from build123d import *

# Parameters (mm, degrees)
SKETCH1_R           = 10
SKETCH1_R_2         = 40
BOSS_EXTRUDE1_DEPTH = 20
SKETCH2_W           = 119.888
SKETCH2_H           = 160
BOSS_EXTRUDE3_DEPTH = 5.08
SKETCH2_7_R         = 29.972
CUT_EXTRUDE1_DEPTH  = 257.843634424
FILLET1_R           = 9.906
FILLET2_R           = 9.906
BOSS_EXTRUDE4_DEPTH = 25.4
BOSS_EXTRUDE5_DEPTH = 25.4


with BuildPart() as part:
    # Sketch1 → Boss-Extrude1 (new body)
    with BuildSketch(Plane.XY.offset(20)):
        with BuildLine():
            Line((95, 80), (-95, 80))
            ThreePointArc((-95, 80), (-98.535533906, 78.535533906), (-100, 75))
            Line((-100, 75), (-100, -75))
            ThreePointArc((-100, -75), (-98.535533906, -78.535533906), (-95, -80))
            Line((-95, -80), (95, -80))
            Line((95, -80), (100, -80))
            Line((100, -80), (100, -75))
            Line((100, -75), (100, 75))
            Line((100, 75), (100, 80))
            Line((100, 80), (95, 80))
        make_face()
        with Locations(Location((-77.895356155, 62.316284924, 0), (0, 0, 180))):
            Circle(SKETCH1_R, mode=Mode.SUBTRACT)
        with Locations(Location((83.46, 0.37, 0), (0, 0, 180))):
            Circle(SKETCH1_R, mode=Mode.SUBTRACT)
        with Locations(Location((-77.895356155, -62.316284924, 0), (0, 0, 180))):
            Circle(SKETCH1_R, mode=Mode.SUBTRACT)
        with Locations(Location((0, 0, 0), (0, 0, 180))):
            Circle(SKETCH1_R_2, mode=Mode.SUBTRACT)
    extrude(amount=-BOSS_EXTRUDE1_DEPTH)

    # Sketch2 → Boss-Extrude3 (add)
    with BuildSketch(Plane(origin=(100, 0, 0), x_dir=(0, 0, -1), z_dir=(1, 0, 0))):
        with Locations((-79.944, 0)):
            Rectangle(SKETCH2_W, SKETCH2_H)
    extrude(amount=-BOSS_EXTRUDE3_DEPTH)

    # Sketch2_7 → Cut-Extrude1 (cut, through all)
    with BuildSketch(Plane(origin=(100, 0, 0), x_dir=(0, 0, -1), z_dir=(1, 0, 0))):
        with Locations((-100.01, 0)):
            Circle(SKETCH2_7_R)
    extrude(amount=-CUT_EXTRUDE1_DEPTH, mode=Mode.SUBTRACT)

    # Fillet1
    fillet1_edges = [part.edges().sort_by_distance(p)[0] for p in [
        (97.46, 80, 139.888),
    ]]
    fillet(fillet1_edges, radius=FILLET1_R)

    # Fillet2
    fillet2_edges = [part.edges().sort_by_distance(p)[0] for p in [
        (97.46, -80, 139.888),
    ]]
    fillet(fillet2_edges, radius=FILLET2_R)

    # Sketch4 → Boss-Extrude4 (add)
    with BuildSketch(Plane.XZ.offset(80)):
        Polygon((94.92, 129.982), (94.92, 20), (-65.1, 20), align=None)
        Polygon((82.22, 32.7), (-24.200327544, 32.7), (82.22, 105.842860042), align=None, mode=Mode.SUBTRACT)
    extrude(amount=-BOSS_EXTRUDE4_DEPTH)

    # Sketch5 → Boss-Extrude5 (add)
    with BuildSketch(Plane(origin=(0, 80, 0), x_dir=(1, 0, 0), z_dir=(0, 1, 0))):
        Polygon((94.92, -129.982), (94.92, -20), (-65.1, -20), align=None)
        Polygon((-24.200327544, -32.7), (82.22, -105.842860042), (82.22, -32.7), align=None, mode=Mode.SUBTRACT)
    extrude(amount=-BOSS_EXTRUDE5_DEPTH)


solid = part.part
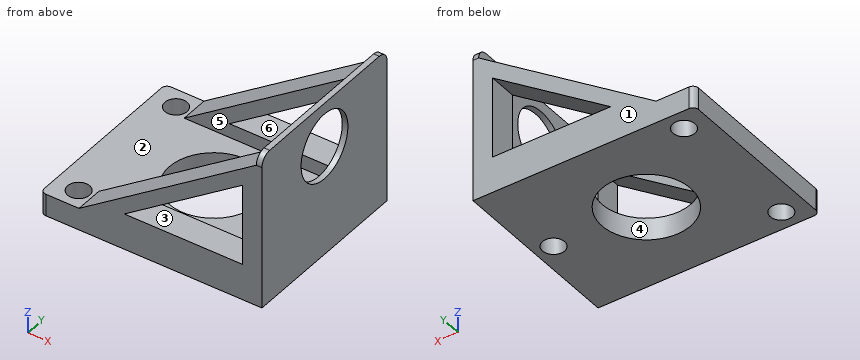
Build history of the part. All positions in model axes, mm. Face numbers are marked on the shaded views. A direction names the side the tool comes from. Give positions to 0.01 mm unless a question says otherwise; leave off trailing zeros. Write each loop counter-clockwise with the first axis right and the second up, starting at its lowest first coordinate (ties: lowest second). Pieces come first, ordered by that corner, then holes. Notation, with made-up numbers: (19, -8.5) - (64, -8.5) arc R17 cw to (64, 22.5) - close; hole circle Ø9 at (-23, -9). An arc over 180 degrees is marked (long way). Use one line per item in the form item = value. Start each with the question number.
1. Band-saw the part on A-A on y = -15. Write the cut outline in (x, z).
2. Two-plate mould, pull along Y, no slides. Class the marked faces 1, 2 and 3: released by +Y, released by -Y, zero draft, split by the parting line, or undercut.
3. Band-saw the part on B-B on x = -31.5. Write the cut outline in (y, z), plus the area to 3 significant figures.
4. Drop flat-ended pins along their axis: pin 1 Ø20.5 at (y, z) = (66, 52) entering from -X; pin 2 Ø1 at (y, z) = (19.5, 27.5) entering from -X; pin 3 Ø20.5 at (x, y) = (14, 67.5) entering from +Z. Give the stop position or say it passes through.
5. Band-saw the part on C-C on z = 45. Write the cut outline in (x, y).
6. Band-saw the part on D-D on z = 91.5. Write the cut outline in (x, y).
7. 3-axis set-ups, long thin cutter, end or side, ignore diameter. For the marked faces 4, 5 and 6: which of +Z, -Z, +X, -X, +Y, -Y reach the whole face in a straight line?
8. Probe line 1 (Y direction, x = -33, z = 34.5); line 2 (Y direction, x = 83, z = 7); line 3 (Z direction, x = -37.5, y = 45). List the from-to ranges inside material, lowest first. Write a range as [from, to].
Conclusion:
q1.outline = (-100, 0) - (-37.08, 0) - (-37.08, 20) - (-100, 20) - close; (37.08, 0) - (100, 0) - (100, 74.06) - (94.92, 74.06) - (94.92, 20) - (37.08, 20) - close; (94.92, 125.96) - (100, 125.96) - (100, 139.89) - (94.92, 139.89) - close
q2.face_1 = released by +Y
q2.face_2 = undercut
q2.face_3 = zero draft
q3.outline = (-80, 0) - (-24.65, 0) - (-24.65, 20) - (-54.6, 20) - (-54.6, 43.09) - (-80, 43.09) - close; (24.65, 0) - (80, 0) - (80, 43.09) - (54.6, 43.09) - (54.6, 20) - (24.65, 20) - close
q3.area = 3,390 mm²
q4.pin_1 = -33.45
q4.pin_2 = 94.92
q4.pin_3 = 81.41
q5.outline = (-28.73, -80) - (-6.3, -80) - (-6.3, -54.6) - (-28.73, -54.6) - close; (-28.73, 54.6) - (-6.3, 54.6) - (-6.3, 80) - (-28.73, 80) - close; (82.22, -80) - (100, -80) - (100, 80) - (82.22, 80) - (82.22, 54.6) - (94.92, 54.6) - (94.92, -54.6) - (82.22, -54.6) - close
q6.outline = (38.93, -80) - (61.35, -80) - (61.35, -54.6) - (38.93, -54.6) - close; (38.93, 54.6) - (61.35, 54.6) - (61.35, 80) - (38.93, 80) - close; (82.22, -80) - (100, -80) - (100, -28.74) - (94.92, -28.74) - (94.92, -54.6) - (82.22, -54.6) - close; (82.22, 54.6) - (94.92, 54.6) - (94.92, 28.74) - (100, 28.74) - (100, 80) - (82.22, 80) - close
q7.face_4 = +Z, -Z
q7.face_5 = +Z, -X
q7.face_6 = +Y, -Y
q8.line_1 = [-80, -54.6], [54.6, 80]
q8.line_2 = [-80, -9.62], [10.36, 80]
q8.line_3 = [0, 20]
